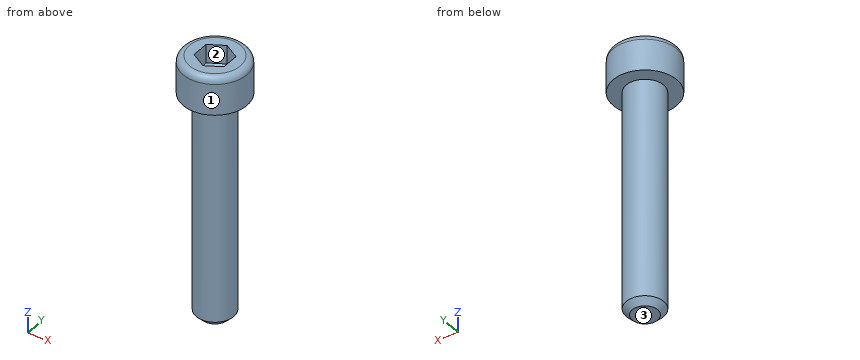
Solid Edge part; units mm, degrees
sketch "Sketch1" plane through (0, 0, 0) normal (0, -1, 0) x (1, 0, 0)
  line L0 (0, 0) -> (3.4, 0)
  arc A0 (3.4, 0) -> (4.25, -0.85) centre (3.4, -0.85) cw
  line L1 (4.25, -0.85) -> (4.25, -5)
  line L2 (4.25, -5) -> (2.5, -5)
  line L3 (2.5, -5) -> (2.5, -34.2)
  line L4 (2.5, -34.2) -> (1.7, -35)
  line L5 (1.7, -35) -> (0, -35)
revolve "RevolvedProtrusion1" add sketch "Sketch1" angle 360 about axis through (0, 0, -35) along (0, 0, 1)
sketch "Sketch2" plane through (0, 0, 0) normal (0, 0, 1) x (1, 0, 0)
  line L0 (-2, -1.1547) -> (-2, 1.1547)
  line L1 (-2, 1.1547) -> (0, 2.3094)
  line L2 (0, 2.3094) -> (2, 1.1547)
  line L3 (2, 1.1547) -> (2, -1.1547)
  line L4 (2, -1.1547) -> (0, -2.3094)
  line L5 (0, -2.3094) -> (-2, -1.1547)
extrude "Cutout1" cut sketch "Sketch2" against normal blind 2.5
sketch "Sketch3" plane through (0, 0, 0) normal (1, 0, 0) x (0, 1, 0)
  line L0 (0, -3.8333) -> (2.3094, -2.5)
  line L1 (0, -2.5) -> (2.3094, -2.5)
  line L2 (0, -2.5) -> (0, -3.8333)
revolve "RevolvedCutout1" cut sketch "Sketch3" angle 360 about axis through (0, 0, -60.325) along (0, 0, 1)
cosmetic_thread "Thread1"
properties part number "21"
Here's how the part is built. I have some questions about the finished solid (model axes, mm). Face numbers are marked on the shaded views. Round coordinates to 2 decimals unless told otherwise and drop trailing zeros. Order: outer loops, then holes, each group sorted by start corner. A loop starts at its lowest first (then second) coordinate and runs counter-clockwise, first axis right, second up. Notation, with made-up numbers: M 87,-16.75 L 135,-16.75 A29 cw 135,14.25 Z; hole C 29.25,13.5 d5. An arc over 180 degrees is marked long. One line per question, with ' | ' between items.
1) I want a section at A-A, the plane z = -18.5. Write out the boundary of the cut face in (x, y).
Working result:
outline: C 0,0 d5
2) For pin 1 Ø2.5 at (y, z) = (-0.5, -1.5) entering from +X; pin 2 Ø0.9 at (x, y) = (-1.5, -2) entering from -Z; pin 3 Ø0.6 at (x, y) = (-0.5, 2) entering from -Z; pin 4 Ø1 at (y, z) = (0, -23) entering from +X, each with a flat end and sliding along its axis, tell me the tip position at first contact or that it passes through.
Working result:
pin 1: x = 4.25 | pin 2: z = -34.65 | pin 3: z = -34.94 | pin 4: x = 2.5
3) I need wall thicknesses on line 1 along Z through (x, y) = (-2.75, 1.75); line 2 along X through (y, z) = (1.5, -33); line 3 along X through (y, z) = (-1.25, -26.5). Which ranges of each line are inside material? Lowest first, please.
Working result:
line 1: -5 to 0 | line 2: -2 to 2 | line 3: -2.17 to 2.17
4) If we mould it in two halves opening along Y, with no side actions, what happens to the marked faces 1, 2 and 3? For each: +Y half, -Y half, draft (parallel to the pull), parting line (faces both ways), or undercut.
Working result:
face 1: parting line | face 2: undercut | face 3: draft
